```python
from build123d import *

# Parameters (mm, degrees)
BASPROSKE_W         = 8
BASPROSKE_H         = 16.5
TOOTHCUT_DEPTH      = 25.667792767
TEETHCUTS_COUNT     = 20
TEETHCUTS_ANGLE     = 342
BORSKE_R            = 3
BORE_DEPTH          = 50.0000508
SKETCH1_R           = 6
BOSS_EXTRUDE1_DEPTH = 6
SKETCH2_R           = 3
CUT_EXTRUDE1_DEPTH  = 6


with BuildPart() as part:
    # BasProSke → Base-Revolve (revolve)
    with BuildSketch(Plane(origin=(0, 0, 0), x_dir=(1, 0, 0), z_dir=(0, 1, 0)), mode=Mode.PRIVATE) as base_revolve_sk:
        with Locations((4, 8.25)):
            Rectangle(BASPROSKE_W, BASPROSKE_H)
    revolve(base_revolve_sk.sketch.rotate(Axis((-10, 0, 0), (1, 0, 0)), 180), axis=Axis((-10, 0, 0), (1, 0, 0)))

    # TooCutSke → ToothCut (cut, through all)
    with BuildSketch(Plane(origin=(0, 0, 0), x_dir=(0, 0, -1), z_dir=(1, 0, 0))):
        with BuildLine():
            ThreePointArc((0.74381438, 13.102904875), (0, 13.124), (-0.74381438, 13.102904875))
            ThreePointArc((-0.74381438, 13.102904875), (-1.226473103, 14.852072512), (-2.209965745, 16.376962373))
            ThreePointArc((-2.209965745, 16.376962373), (0, 16.5254), (2.209965745, 16.376962373))
            ThreePointArc((2.209965745, 16.376962373), (1.226473103, 14.852072512), (0.74381438, 13.102904875))
        make_face()
    toothcut = extrude(amount=TOOTHCUT_DEPTH, mode=Mode.SUBTRACT)

    # TeethCuts: ToothCut ×20 about axis
    teethcuts_axis = Axis((-10, 0, 0), (1, 0, 0))
    for i in range(1, TEETHCUTS_COUNT):
        add(toothcut.rotate(teethcuts_axis, i * TEETHCUTS_ANGLE / (TEETHCUTS_COUNT - 1)), mode=Mode.SUBTRACT)

    # BorSke → Bore (cut, symmetric)
    with BuildSketch(Plane(origin=(0, 0, 0), x_dir=(0, 0, -1), z_dir=(1, 0, 0))):
        with Locations(Location((0, 0, 0), (0, 0, 180))):
            Circle(BORSKE_R)
    extrude(amount=BORE_DEPTH, both=True, mode=Mode.SUBTRACT)

    # Sketch1 → Boss-Extrude1 (add)
    with BuildSketch(Plane(origin=(8, 0, 0), x_dir=(0, 0, -1), z_dir=(1, 0, 0))):
        with Locations(Location((0, 0, 0), (0, 0, 180))):
            Circle(SKETCH1_R)
    extrude(amount=BOSS_EXTRUDE1_DEPTH)

    # Sketch2 → Cut-Extrude1 (cut)
    with BuildSketch(Plane(origin=(14, 0, 0), x_dir=(0, 0, -1), z_dir=(1, 0, 0))):
        Circle(SKETCH2_R)
    extrude(amount=-CUT_EXTRUDE1_DEPTH, mode=Mode.SUBTRACT)


solid = part.part
```
Could you check a few things on this model? Use its own coordinates, in mm. A direction names the side the tool comes from. Coordinates: 2 decimals unless noted, no trailing zeros. Write each loop counter-clockwise with the first axis right and the second up, starting at its lowest first coordinate (ties: lowest second). Pieces come first, ordered by that corner, then holes. Notation, with made-up numbers: (76, 48) -> (87, 48) arc R29 ccw to (87, 77) -> close; hole circle Ø4 at (-12, 12.25). An arc over 180 degrees is marked (long way). Write item = value, one per line. Start each with the question number.
(1) We'd pull the mould along Y, two halves only. Please class faces 5 (the face through (0, -0.2, -3.4)), 6 (the face through (4, 14, -6)), 7 (the face through (3.94, 12.75, 7.74)), 8 (the face through (3.944, -11.274, -9.687)): released by +Y, released by -Y, zero draft, split by the parting line, or undercut.
(2) I want a section at C-C (x = 13). Please give me the cut outline in (y, z), plus the area to 3 significant figures.
(3) Which directions (+Z, -Z, +X, -X, +Y, -Y) give clear straight access to the entire face, cutting with the end or side of a thin tool? Please do faces 1 (the face through (4, -6, 14)), 2 (the face through (3.944, 1.21, -14.815)), 3 (the face through (10.958, -1.802, 5.723)), 4 (the face through (3.944, -3.427, -14.464)).
(4) I need wall thicknesses on line 1 (Y direction, x = 5, z = 0); line 2 (Z direction, x = 6, y = 14); line 3 (Z direction, x = 2.25, y = -13). Which ranges of each line are inside material? Lowest first, please. Write a range as [from, to].
(5) I want a section at A-A (y = 0). Please give me the cut outline in (x, z), plus the area to 3 significant figures.
(6) Will these pins go through, and if not, where does the flat tip stop? pin 1 (5 mm diameter, centred on y = 10, z = -2, fed in from -X); pin 2 (6 mm diameter, centred on x = 11.5, z = -5, fed in from -Y); pin 3 (8 mm diameter, centred on x = 3, y = -5.5, fed in from -Z); pin 4 (5.5 mm diameter, centred on y = 0, z = 0, fed in from -X).
Result set:
q1.face_5 = zero draft
q1.face_6 = released by +Y
q1.face_7 = undercut
q1.face_8 = released by -Y
q2.outline = circle Ø12 at (0, 0); hole circle Ø6 at (0, 0)
q2.area = 84.8 mm2
q3.face_1 = +Z, +X, -X
q3.face_2 = -Z, +X, -X
q3.face_3 = +X
q3.face_4 = +X, -X
q4.line_1 = [-13.12, -3], [3, 13.12]
q4.line_2 = [-7.87, -6], [-3.46, -0.92], [0.92, 3.46], [6, 7.87]
q4.line_3 = [-7.79, -5.18], [-3.39, 3.39], [5.18, 7.79]
q5.outline = (0, -13.12) -> (8, -13.12) -> (8, -6) -> (14, -6) -> (14, -3) -> (0, -3) -> close; (0, 3) -> (14, 3) -> (14, 6) -> (8, 6) -> (8, 13.12) -> (0, 13.12) -> close
q5.area = 198 mm2
q6.pin_1 = 0
q6.pin_2 = -5.66
q6.pin_3 = -16.35
q6.pin_4 = through
